Autodesk Inventor part; units mm, degrees
ref_plane "YZ Plane" through (0, 0, 0) normal (1, 0, 0) x (0, 1, 0)
ref_plane "XZ Plane" through (0, 0, 0) normal (0, 1, 0) x (-1, 0, 0)
ref_plane "XY Plane" through (0, 0, 0) normal (0, 0, 1) x (1, 0, 0)
sketch "スケッチ1" plane through (0, 0, 0) normal (1, 0, 0) x (0, 1, 0)
  circle A0 centre (0, 0) radius 16.5
  dimension "d0" = 33
extrude "押し出し1" add sketch "スケッチ1" along normal blind 25.5
sketch "スケッチ2" plane through (25.5, 0, 0) normal (1, 0, 0) x (0, 0, -1)
  circle A0 centre (0, 0) radius 20
  dimension "d3" = 40
extrude "押し出し2" add sketch "スケッチ2" along normal blind 1
sketch "スケッチ3" plane through (0, 0, 0) normal (-1, 0, 0) x (0, 0, 1)
  circle A0 centre (0, 0) radius 20
  dimension "d6" = 40
extrude "押し出し3" add sketch "スケッチ3" along normal blind 1
sketch "スケッチ4" plane through (26.5, 0, 0) normal (1, 0, 0) x (0, 0, -1)
  circle A0 centre (0, 0) radius 5.5
  dimension "d9" = 11
extrude "押し出し4" add sketch "スケッチ4" along normal blind 2
sketch "スケッチ5" plane through (-1, 0, 0) normal (-1, 0, 0) x (0, 0, 1)
  circle A0 centre (0, 0) radius 5.5
  dimension "d12" = 11
extrude "押し出し5" add sketch "スケッチ5" along normal blind 2
sketch "スケッチ6" plane through (28.5, 0, 0) normal (1, 0, 0) x (0, 0, -1)
  circle A0 centre (0, 0) radius 5.5
hole "穴1" at (28.5, 0, 0) direction (-1, 0, 0) diameter 6.1 end through all
properties part number "CLS_24.5N" material "ポリプロピレン"
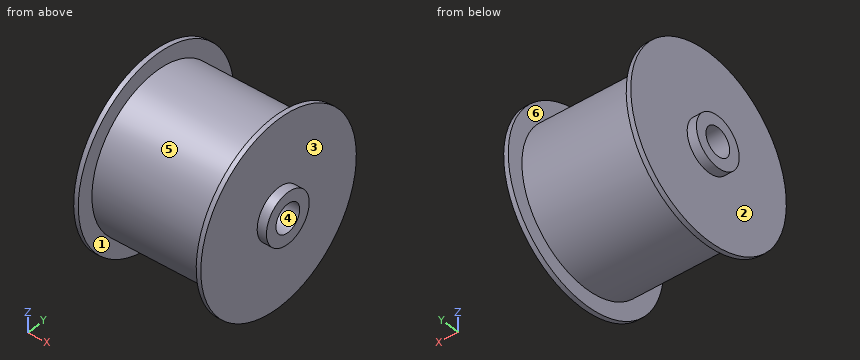
Model file for the job. Use its own axes, mm. Face numbers are marked on the shaded views. A direction names the side the tool comes from. Coordinates: 2 decimals unless noted, no trailing zeros. Loops run counter-clockwise (first coordinate to the right, second up) from the corner with the lowest first, then second, coordinate; pieces in that order, holes last. Notation, with made-up numbers: (27.25, 35.5) - (86.25, 35.5) arc R25 ccw to (86.25, 61.5) - close; hole circle Ø9 at (-16.75, 5.5). An arc over 180 degrees is marked (long way). Write item = value, one per line. Start each with the question number.
Item 1: Drop flat-ended pins along their axis: pin 1 Ø12 at (y, z) = (-8, 1.5) entering from +X; pin 2 Ø1 at (x, z) = (12, 9) entering from +Y; pin 3 Ø6 at (x, z) = (11, -9.5) entering from -Y; pin 4 Ø10 at (y, z) = (-12, 14) entering from -X. Give the stop position or say it passes through.
Item 2: Saw through at A-A, the plane z = 0. List the corners of the cut face in (x, y).
Item 3: Wall check: probe 1 along Z at (x, y) = (18, 0); probe 2 along X at (y, z) = (4, 17.5); probe 3 along X at (y, z) = (3, -14.5). Give the ranges that are in metal, low to high. Write a range as [from, to].
Item 4: Saw through at D-D, the plane z = 8. List the corners of the cut face in (x, y).
Item 5: Pull direction Z, two halves, no side cores. Call the marked faces 4, 5 and 6: +Z half, -Z half, draft (parallel to the pull), parting line (faces both ways), or undercut.
Item 6: 3-axis set-ups, long thin cutter, end or side, ignore diameter. For the marked faces 1, 2 and 3: which of +Z, -Z, +X, -X, +Y, -Y reach the whole face in a straight line?
Item 7: Saw through at C-C, the plane x = 10.5. List the corners of the cut face in (y, z).
Answers:
q1.pin_1 = 28.5
q1.pin_2 = 14.14
q1.pin_3 = -15.17
q1.pin_4 = -1
q2.outline = (-3, -5.5) - (-1, -5.5) - (-1, -20) - (0, -20) - (0, -16.5) - (25.5, -16.5) - (25.5, -20) - (26.5, -20) - (26.5, -5.5) - (28.5, -5.5) - (28.5, -3.05) - (-3, -3.05) - close; (-3, 3.05) - (28.5, 3.05) - (28.5, 5.5) - (26.5, 5.5) - (26.5, 20) - (25.5, 20) - (25.5, 16.5) - (0, 16.5) - (0, 20) - (-1, 20) - (-1, 5.5) - (-3, 5.5) - close
q3.probe_1 = [-16.5, -3.05], [3.05, 16.5]
q3.probe_2 = [-1, 0], [25.5, 26.5]
q3.probe_3 = [-1, 26.5]
q4.outline = (-1, -18.33) - (0, -18.33) - (0, -14.43) - (25.5, -14.43) - (25.5, -18.33) - (26.5, -18.33) - (26.5, 18.33) - (25.5, 18.33) - (25.5, 14.43) - (0, 14.43) - (0, 18.33) - (-1, 18.33) - close
q5.face_4 = undercut
q5.face_5 = parting line
q5.face_6 = draft
q6.face_1 = none
q6.face_2 = -X
q6.face_3 = +X
q7.outline = circle Ø33 at (0, 0); hole circle Ø6.1 at (0, 0)
